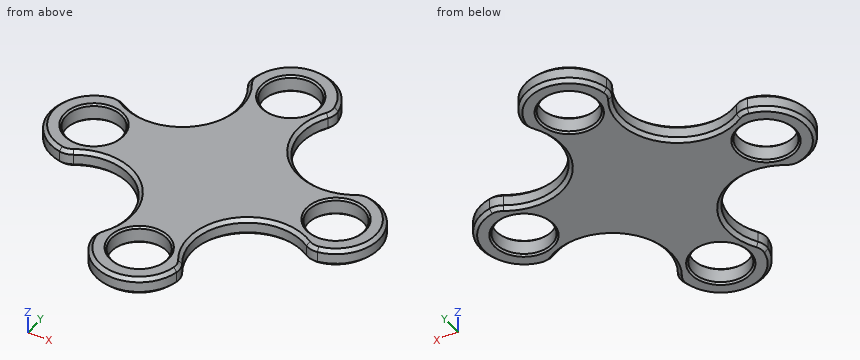
from build123d import *

# Parameters (mm, degrees)
F0_R     = 8
F1_DEPTH = 5
F2_SIZE  = 1
F3_SIZE  = 0.5


# Not quite as in the source:
# - a feature names something its author has since deleted; it is built from what else it names


with BuildPart() as f1:
    # F0 (on Top) → F1 (new body)
    with BuildSketch(Plane.XY):
        with BuildLine():
            ThreePointArc((11.6083434008, 33.7208583728), (12.2845984061, 35.4442804748), (12.2873952004, 37.2956304556))
            ThreePointArc((12.2873952004, 37.2956304556), (0, 47.5), (-12.2873952004, 37.2956304556))
            ThreePointArc((-12.2873952004, 37.2956304556), (-12.2845984061, 35.4442804748), (-11.6083434008, 33.7208583728))
            ThreePointArc((-11.6083434008, 33.7208583728), (-13.8553017596, 13.8553017596), (-33.7208583728, 11.6083434008))
            ThreePointArc((-33.7208583728, 11.6083434008), (-35.4442804748, 12.2845984061), (-37.2956304556, 12.2873952004))
            ThreePointArc((-37.2956304556, 12.2873952004), (-47.5, 0), (-37.2956304556, -12.2873952004))
            ThreePointArc((-37.2956304556, -12.2873952004), (-35.4442804748, -12.2845984061), (-33.7208583728, -11.6083434008))
            ThreePointArc((-33.7208583728, -11.6083434008), (-13.8553017596, -13.8553017596), (-11.6083434008, -33.7208583728))
            ThreePointArc((-11.6083434008, -33.7208583728), (-12.2845984061, -35.4442804748), (-12.2873952004, -37.2956304556))
            ThreePointArc((-12.2873952004, -37.2956304556), (0, -47.5), (12.2873952004, -37.2956304556))
            ThreePointArc((12.2873952004, -37.2956304556), (12.2845984061, -35.4442804748), (11.6083434008, -33.7208583728))
            ThreePointArc((11.6083434008, -33.7208583728), (13.8553017596, -13.8553017596), (33.7208583728, -11.6083434008))
            ThreePointArc((33.7208583728, -11.6083434008), (35.4442804748, -12.2845984061), (37.2956304556, -12.2873952004))
            ThreePointArc((37.2956304556, -12.2873952004), (47.5, 0), (37.2956304556, 12.2873952004))
            ThreePointArc((37.2956304556, 12.2873952004), (35.4442804748, 12.2845984061), (33.7208583728, 11.6083434008))
            ThreePointArc((33.7208583728, 11.6083434008), (13.8553017596, 13.8553017596), (11.6083434008, 33.7208583728))
        make_face()
        with Locations((0, -35)):
            Circle(F0_R, mode=Mode.SUBTRACT)
        with Locations((-35, 0)):
            Circle(F0_R, mode=Mode.SUBTRACT)
        with Locations((35, 0)):
            Circle(F0_R, mode=Mode.SUBTRACT)
        with Locations((0, 35)):
            Circle(F0_R, mode=Mode.SUBTRACT)
    extrude(amount=F1_DEPTH)

    # F2
    f2_edges = [f1.edges().sort_by_distance(p)[0] for p in [
        (-47.5, 0, 5),
        (-13.855302, -13.855302, 5),
        (-13.855302, 13.855302, 5),
        (0, 47.5, 5),
        (13.855302, 13.855302, 5),
        (47.5, 0, 5),
        (13.855302, -13.855302, 5),
        (0, -47.5, 5),
        (13.855302, 13.855302, 0),
        (0, 47.5, 0),
        (-13.855302, 13.855302, 0),
        (-47.5, 0, 0),
        (-13.855302, -13.855302, 0),
        (0, -47.5, 0),
        (13.855302, -13.855302, 0),
        (47.5, 0, 0),
    ]]
    chamfer(f2_edges, length=F2_SIZE)

    # F3
    f3_edges = [f1.edges().sort_by_distance(p)[0] for p in [
        (-8, 35, 5),
        (-8, -35, 5),
        (27, 0, 5),
        (-43, 0, 5),
        (-8, 35, 0),
        (-43, 0, 0),
        (27, 0, 0),
        (-8, -35, 0),
    ]]
    chamfer(f3_edges, length=F3_SIZE)


solid = f1.part
Part model, mm, in its own coordinate system. Give positions to 0.01 mm unless a question says otherwise; leave off trailing zeros. Order: outer loops, then holes, each group sorted by start corner. A loop starts at its lowest first (then second) coordinate and runs counter-clockwise, first axis right, second up. Notation, with made-up numbers: (23, 34.5) - (44, 34.5) arc R15 ccw to (44, 53.5) - close; hole circle Ø6 at (67, 15.5). An arc over 180 degrees is marked (long way). One line per question, with ' | ' between items.
1. Band-saw the part on A-A on y = 0. List the corners of the cut face in (x, z), then the cut area to 3 significant figures.
Filled in:
outline: (-47.5, 1) - (-46.5, 0) - (-43.5, 0) - (-43, 0.5) - (-43, 4.5) - (-43.5, 5) - (-46.5, 5) - (-47.5, 4) - close; (-27, 0.5) - (-26.5, 0) - (26.5, 0) - (27, 0.5) - (27, 4.5) - (26.5, 5) - (-26.5, 5) - (-27, 4.5) - close; (43, 0.5) - (43.5, 0) - (46.5, 0) - (47.5, 1) - (47.5, 4) - (46.5, 5) - (43.5, 5) - (43, 4.5) - close | area: 312 mm²
2. Drop a flat-ended pin along its axis: P1, Ø3, axis at x = 33, z = 1.5, coming from the +Y side. Give the stop position or say it passes through.
Filled in:
P1: y = 12.01
3. Drill centre lines: probe 1 along Y at (x, z) = (0, 1.65); probe 2 along Y at (x, z) = (1, 1.6); probe 3 along Y at (x, z) = (-32, 4.25). Where is each one in solid material? Low to high.
Filled in:
probe 1: -47.5 to -43, -27 to 27, 43 to 47.5 | probe 2: -47.46 to -42.94, -27.06 to 27.06, 42.94 to 47.46 | probe 3: -10.39 to -7.42, 7.42 to 10.39
4. Band-saw the part on B-B on z = 2.45. List the corners of the cut face in (x, y).
Filled in:
outline: (-37.3, -12.29) arc R5 ccw to (-33.72, -11.61) arc R16.04 cw to (-11.61, -33.72) arc R5 ccw to (-12.29, -37.3) arc R12.5 ccw to (12.29, -37.3) arc R5 ccw to (11.61, -33.72) arc R16.04 cw to (33.72, -11.61) arc R5 ccw to (37.3, -12.29) arc R12.5 ccw to (37.3, 12.29) arc R5 ccw to (33.72, 11.61) arc R16.04 cw to (11.61, 33.72) arc R5 ccw to (12.29, 37.3) arc R12.5 ccw to (-12.29, 37.3) arc R5 ccw to (-11.61, 33.72) arc R16.04 cw to (-33.72, 11.61) arc R5 ccw to (-37.3, 12.29) arc R12.5 ccw to start; hole circle Ø16 at (-35, 0); hole circle Ø16 at (0, -35); hole circle Ø16 at (0, 35); hole circle Ø16 at (35, 0)
